Solid Edge part; units mm, degrees
sketch "Sketch1" plane through (0, 0, 0) normal (0, -1, 0) x (1, 0, 0)
  circle A0 centre (0, 0) radius 10.5
extrude "Protrusion1" add sketch "Sketch1" along normal mid plane 4
hole "Bohrung_1" at (0, -2, 0) direction (0, 1, 0) diameter 15 end up to next
fillet "Verrundung_1" radius 0.5 4 edges at (-10.5, -2, 0) (-10.5, 2, 0) (-7.5, -2, 0) (0, 2, -7.5)
properties material "Aluminium, 1060"
Read the model definition and answer for the solid it produces. Units are mm, in the model's axes. Round coordinates to 2 decimals unless told otherwise and drop trailing zeros. Write each loop counter-clockwise with the first axis right and the second up, starting at its lowest first coordinate (ties: lowest second). Pieces come first, ordered by that corner, then holes. Notation, with made-up numbers: M 63,77.5 L 82,77.5 A20 ccw 82,90.5 Z; hole C 5.25,51.5 d10. An arc over 180 degrees is marked long. One line per item, written item: value.
Q1. Find section A-A on x = 0. Write down the section's boundary in (y, z).
Data:
outline: M -2,-10 A0.5 ccw -1.5,-10.5 L 1.5,-10.5 A0.5 ccw 2,-10 L 2,-8 A0.5 ccw 1.5,-7.5 L -1.5,-7.5 A0.5 ccw -2,-8 Z; M -2,8 A0.5 ccw -1.5,7.5 L 1.5,7.5 A0.5 ccw 2,8 L 2,10 A0.5 ccw 1.5,10.5 L -1.5,10.5 A0.5 ccw -2,10 Z
Q2. Find section C-C on y = -0.25. Write down the section's boundary in (x, z), plus the area to 3 significant figures.
Data:
outline: C 0,0 d21; hole C 0,0 d15
area: 170 mm2
Q3. Find section B-B on z = 0. Write down the section's boundary in (x, y).
Data:
outline: M -10.5,-1.5 A0.5 ccw -10,-2 L -8,-2 A0.5 ccw -7.5,-1.5 L -7.5,1.5 A0.5 ccw -8,2 L -10,2 A0.5 ccw -10.5,1.5 Z; M 7.5,-1.5 A0.5 ccw 8,-2 L 10,-2 A0.5 ccw 10.5,-1.5 L 10.5,1.5 A0.5 ccw 10,2 L 8,2 A0.5 ccw 7.5,1.5 Z
Q4. Straight lines are drawn through the part: line 1 (Z direction, x = 0, y = 0.2); line 2 (X direction, y = -1.3, z = 4.25); line 3 (Z direction, x = 4.5, y = -0.45). For each, find the intervals that lie inside material, in ascending order. Write a range as [from, to].
Data:
line 1: [-10.5, -7.5], [7.5, 10.5]
line 2: [-9.6, -6.18], [6.18, 9.6]
line 3: [-9.49, -6], [6, 9.49]
Q5. Flat-ended cylindrical pins translate along their axes: pin 1 Ø2 at (y, z) = (1, -3) entering from +X; pin 2 Ø1 at (x, y) = (3, 0.5) entering from +Z. Find the tip coordinate at first contact, or state that the pin passes through.
Data:
pin 1: x = 10.31
pin 2: z = 10.2
Q6. For a pull along X with two mould halves and no side action, classify faces 1 (the cylindrical face through (10, 0, 3.2)), 2 (the flat face through (8.2, -2, 0)), 3 (the cylindrical face through (0.33, -0.021, 7.493)) as +X half, -X half, draft (parallel to the pull), parting line (faces both ways), or undercut.
Data:
face 1: parting line
face 2: draft
face 3: undercut
